from build123d import *

# Parameters (mm, degrees)
SKETCH1_W             = 26
SKETCH1_H             = 12
BOSS_EXTRUDE1_DEPTH   = 40
SKETCH2_W             = 10
SKETCH2_H             = 40
BOSS_EXTRUDE2_DEPTH   = 48
CUT_EXTRUDE1_DEPTH    = 48
M3_TAPPED_HOLE1_D     = 2.5
M3_TAPPED_HOLE1_DEPTH = 6
M3_TAPPED_HOLE1_TIP   = 0.751075774
M4_TAPPED_HOLE1_D     = 3.3
M4_TAPPED_HOLE1_DEPTH = 8
M4_TAPPED_HOLE1_TIP   = 0.991420021
CHAMFER1_SIZE         = 0.5


with BuildPart() as part:
    # Sketch1 → Boss-Extrude1 (new body)
    with BuildSketch(Plane.XY):
        with Locations((2.110588235, -0.708235294)):
            Rectangle(SKETCH1_W, SKETCH1_H)
    extrude(amount=BOSS_EXTRUDE1_DEPTH)

    # Sketch2 → Boss-Extrude2 (add)
    with BuildSketch(Plane(origin=(0, 5.291764706, 0), x_dir=(1, 0, 0), z_dir=(0, 1, 0))):
        with Locations((2.110588235, -20)):
            Rectangle(SKETCH2_W, SKETCH2_H)
    extrude(amount=BOSS_EXTRUDE2_DEPTH)

    # Sketch3 → Cut-Extrude1 (cut)
    with BuildSketch(Plane.ZY.offset(2.889411765)):
        Polygon((0, 21.841764706), (3.389763468, 21.841764706), (3.389763468, 23.541764706), (6.66389663, 23.541764706), (6.66389663, 15.541764706), (3.389763468, 15.541764706), (3.389763468, 17.241764706), (0, 17.241764706), align=None)
    extrude(amount=-CUT_EXTRUDE1_DEPTH, mode=Mode.SUBTRACT)

    # M3 Tapped Hole1
    with Locations(Plane(origin=(0, 0, 0), x_dir=(-1, 0, 0), z_dir=(0, 0, -1))):
        with Locations((-9.110588235, -0.708235294), (4.889411765, -0.708235294), (-2.110588235, 51.291764706)):
            Hole(M3_TAPPED_HOLE1_D / 2, depth=M3_TAPPED_HOLE1_DEPTH)
            with Locations((0, 0, -(M3_TAPPED_HOLE1_DEPTH + M3_TAPPED_HOLE1_TIP / 2))):  # 118° drill point
                Cone(0, M3_TAPPED_HOLE1_D / 2, M3_TAPPED_HOLE1_TIP, mode=Mode.SUBTRACT)

    # M4 Tapped Hole1
    with Locations(Plane(origin=(0, 53.291764706, 0), x_dir=(1, 0, 0), z_dir=(0, 1, 0))):
        with Locations((2.110588235, -10), (2.110588235, -30)):
            Hole(M4_TAPPED_HOLE1_D / 2, depth=M4_TAPPED_HOLE1_DEPTH)
            with Locations((0, 0, -(M4_TAPPED_HOLE1_DEPTH + M4_TAPPED_HOLE1_TIP / 2))):  # 118° drill point
                Cone(0, M4_TAPPED_HOLE1_D / 2, M4_TAPPED_HOLE1_TIP, mode=Mode.SUBTRACT)

    # Chamfer1
    chamfer1_edges = [part.edges().sort_by_distance(p)[0] for p in [
        (-2.889411765, 53.291764706, 20),
        (7.110588235, 53.291764706, 20),
    ]]
    chamfer(chamfer1_edges, length=CHAMFER1_SIZE)


solid = part.part
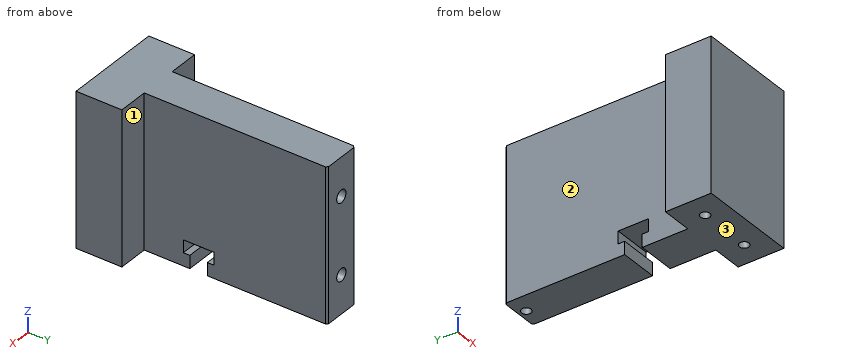
CAD build for the part. Positions are in the model's coordinates, mm. Face numbers are marked on the shaded views. A direction names the side the tool comes from. Coordinates: 2 decimals unless noted, no trailing zeros. Loops run counter-clockwise (first coordinate to the right, second up) from the corner with the lowest first, then second, coordinate; pieces in that order, holes last. Notation, with made-up numbers: (-16.75, 57) - (16.25, 57) arc R17 cw to (16.25, 74) - close; hole circle Ø9 at (38.25, 39.25). An arc over 180 degrees is marked (long way). Write item = value, one per line. Start each with the question number.
Q1. Flat gauge pins, fed straight in: pin 1 Ø12 at (x, z) = (-7, 24.5) entering from +Y; pin 2 Ø20 at (y, z) = (35.5, 15.5) entering from +X; pin 3 Ø5 at (x, z) = (-6, 33) entering from +Y; pin 4 Ø3 at (x, y) = (-5.5, 34.5) entering from -Z. Where does each tip first touch, or does it go through?
Q2. Drill centre lines: L1, parallel to Z at x = 4.25, y = 23; L2, parallel to X at y = 47, z = 30; L3, parallel to Z at x = 6.5, y = 21. Where is each one in solid material? Low to high.
Q3. Cut at A-A, the plane z = 19. List the corners of the cut face in (x, y).
Q4. Cut at B-B, the plane x = -8.25. List the corners of the cut face in (y, z), then the cut area to 3 significant figures.
Q5. Cut at C-C, the plane y = 6. List the corners of the cut face in (x, z).
Q6. Which spindle directions (+Z, -Z, +X, -X, +Y, -Y) get a long thin tool onto all of the face, cutting with end or side? Do the marked faces 1, 2 and 3. Say none if no direction does.
Computed:
q1.pin_1 = 53.29
q1.pin_2 = 7.11
q1.pin_3 = 5.29
q1.pin_4 = through
q2.L1 = 0 to 3.39, 6.66 to 40
q2.L2 = -2.89 to 0.46, 3.76 to 7.11
q2.L3 = 6.66 to 40
q3.outline = (-10.89, -6.71) - (15.11, -6.71) - (15.11, 5.29) - (7.11, 5.29) - (7.11, 52.79) - (6.61, 53.29) - (-2.39, 53.29) - (-2.89, 52.79) - (-2.89, 5.29) - (-10.89, 5.29) - close
q4.outline = (-6.71, 0) - (5.29, 0) - (5.29, 40) - (-6.71, 40) - close
q4.area = 480 mm²
q5.outline = (-2.89, 0) - (7.11, 0) - (7.11, 40) - (-2.89, 40) - close
q6.face_1 = +Z, -Z, +X, +Y
q6.face_2 = +Z, -Z, -X, +Y
q6.face_3 = -Z, +X, -X, +Y, -Y
